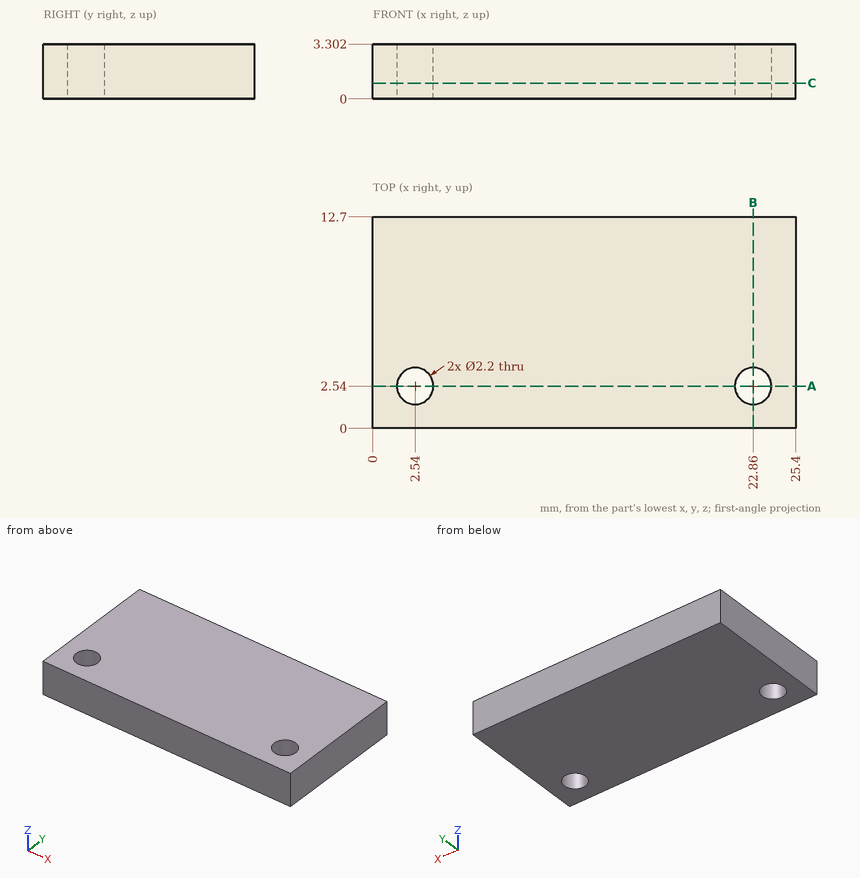
Geometry check sheet. Reference: drawing and pictorial views, mm from the part's lowest x, y, z. Coordinates: 2 decimals unless noted, no trailing zeros. Write each loop counter-clockwise with the first axis right and the second up, starting at its lowest first coordinate (ties: lowest second). Pieces come first, ordered by that corner, then holes. Notation, with made-up numbers: M 52,30.5 L 111,30.5 A9 ccw 111,45.5 Z; hole C -31,-34 d3. An arc over 180 degrees is marked long. Write item = value, one per line. Start each with the question number.
1. Sectioned sample at C-C (z = 0.95). Record the cut outline in (x, y).
2. Sectioned sample at B-B (x = 22.86). Record the cut outline in (y, z), then the cut area to 3 significant figures.
3. Sectioned sample at A-A (y = 2.54). Record the cut outline in (x, z), then the cut area to 3 significant figures.
4. Thickness scan on probe 1 along Y at (x, z) = (22.86, 2.35); probe 2 along Y at (x, z) = (3.25, 1.15). Record the ranges inside material, lowest first.
The answers:
q1.outline = M 0,0 L 25.4,0 L 25.4,12.7 L 0,12.7 Z; hole C 2.54,2.54 d2.2; hole C 22.86,2.54 d2.2
q2.outline = M 0,0 L 1.44,0 L 1.44,3.3 L 0,3.3 Z; M 3.64,0 L 12.7,0 L 12.7,3.3 L 3.64,3.3 Z
q2.area = 34.7 mm²
q3.outline = M 0,0 L 1.44,0 L 1.44,3.3 L 0,3.3 Z; M 3.64,0 L 21.76,0 L 21.76,3.3 L 3.64,3.3 Z; M 23.96,0 L 25.4,0 L 25.4,3.3 L 23.96,3.3 Z
q3.area = 69.3 mm²
q4.probe_1 = 0 to 1.44, 3.64 to 12.7
q4.probe_2 = 0 to 1.7, 3.38 to 12.7
